```python
from build123d import *

# Parameters (mm, degrees)
SKETCH2_R          = 2.25
SKETCH2_R_2        = 2.036849222
CUT_EXTRUDE1_DEPTH = 10
CHAMFER1_SIZE      = 0.5
CHAMFER2_SIZE      = 0.5


with BuildPart() as part:
    # Sketch1 → Revolve1 (revolve)
    with BuildSketch(Plane(origin=(0, 0, 0), x_dir=(1, 0, 0), z_dir=(0, 1, 0))):
        Polygon((-29.626724138, 24.634482759), (-33.376724138, 24.634482759), (-33.376724138, 9.634482759), (-42.126724138, 9.634482759), (-42.126724138, 6.634482759), (-58.126724138, 6.634482759), (-58.126724138, 1.634482759), (-48.626724138, 1.634482759), (-48.626724138, -38.365517241), (-45.626724138, -38.365517241), (-45.626724138, -75.365517241), (-29.626724138, -75.365517241), align=None)
    revolve(axis=Axis((-29.626724138, 0, -29.85316092), (0, 0, 1)))

    # Sketch2 → Cut-Extrude1 (cut)
    with BuildSketch(Plane.XY.offset(-1.634482759)):
        with Locations((-4.626724138, 0)):
            Circle(SKETCH2_R)
        with Locations((-29.626724138, 25)):
            Circle(SKETCH2_R_2)
        with Locations((-54.626724138, 0)):
            Circle(SKETCH2_R)
        with Locations((-29.626724138, -25)):
            Circle(SKETCH2_R)
    extrude(amount=-CUT_EXTRUDE1_DEPTH, mode=Mode.SUBTRACT)

    # Chamfer1
    chamfer1_edges = [part.edges().sort_by_distance(p)[0] for p in [
        (-6.876724138, 0, -6.634482759),
        (-6.876724138, 0, -1.634482759),
        (-31.66357336, 25, -6.634482759),
        (-31.66357336, 25, -1.634482759),
        (-56.876724138, 0, -6.634482759),
        (-56.876724138, 0, -1.634482759),
        (-31.876724138, -25, -6.634482759),
        (-31.876724138, -25, -1.634482759),
        (-25.876724138, 0, -24.634482759),
        (-17.126724138, 0, -9.634482759),
        (-1.126724138, 0, -6.634482759),
        (-1.126724138, 0, -1.634482759),
    ]]
    chamfer(chamfer1_edges, length=CHAMFER1_SIZE)

    # Chamfer2
    chamfer2_edges = [part.edges().sort_by_distance(p)[0] for p in [
        (-10.626724138, 0, 38.365517241),
        (-13.626724138, 0, 75.365517241),
    ]]
    chamfer(chamfer2_edges, length=CHAMFER2_SIZE)


solid = part.part
```
Geometry check sheet. Reference: the model listing, model coordinates, mm. A direction names the side the tool comes from. Round coordinates to 2 decimals unless told otherwise and drop trailing zeros. Loops run counter-clockwise (first coordinate to the right, second up) from the corner with the lowest first, then second, coordinate; pieces in that order, holes last. Notation, with made-up numbers: (-3, 84.25) - (41, 84.25) arc R21 cw to (41, 101.25) - close; hole circle Ø1 at (-8.5, 28). An arc over 180 degrees is marked (long way). Write each question's results on one line, items separated by ' | '. Start each with the question number.
Q1. Cross-section at D-D on z = -13. Enter the section's corners in (x, y).
Q2. Access from +Z, -Z, +X, -X, +Y, -Y to the whole of each face (thin tool, end or side, straight path). Record for faces 4 (the flat face through (-21, -14, 38.366)), 5 (the flat face through (-27, -3, -9.634)), 6 (the cylindrical face through (-56.8, -8.6, -4.1)).
Q3. Gauge pin test, flat ends, axial feed: P1, Ø3, axis at x = -27.5, z = 42.5, coming from the -Y side; P2, Ø1, axis at y = 1, z = -3.5, coming from the +X side; P3, Ø3, axis at x = -48.5, z = -3.5, coming from the +Y side. Record the tip position at first contact, or that the pin passes through.
Q4. Release check for a two-part mould opening along X. For faces 1 (the flat face through (-29, 0, 75.366)), 2 (the cylindrical face through (-33.204, -1.126, -16.783)), 3 (the cylindrical face through (-31.243, 23.761, -4.106)) record: +X half, -X half, draft (parallel to the pull), parting line (faces both ways), or undercut.
Q5. Cross-section at B-B on z = 23. Enter the section's corners in (x, y), and give its area (3 significant figures).
Q6. Thickness scan on line 1 (Z direction, x = -51, y = 5.5); line 2 (Z direction, x = -24, y = 10.5); line 3 (X direction, y = -11, z = 8.5). Record the ranges inside material, lowest first. Write a range as [from, to].
Q7. Cross-section at A-A on y = 0. State how many separate pieces and enclosed holes the cut face has, and give its area (3 significant figures).
Answers below:
1) outline: circle Ø7.5 at (-29.63, 0)
2) face 4: +Z | face 5: -Z | face 6: +Z, -Z
3) P1: stops at y = -15.99 | P2: stops at x = -1.13 | P3: stops at y = 22.59
4) face 1: draft | face 2: parting line | face 3: undercut
5) outline: circle Ø38 at (-29.63, 0) | area: 1,130 mm²
6) line 1: z = [-6.63, -1.63] | line 2: z = [-9.63, 75.37] | line 3: x = [-45.12, -14.13]
7) separate pieces: 3 | enclosed holes: 0 | area: 3,130 mm²
